Design review of the part built by this model. Coordinates are the model's own, in mm. Coordinates: 2 decimals unless noted, no trailing zeros. Order: outer loops, then holes, each group sorted by start corner. A loop starts at its lowest first (then second) coordinate and runs counter-clockwise, first axis right, second up. Notation, with made-up numbers: M 23,-36 L 36,-36 A10 cw 36,-22 Z; hole C 81,23.5 d6. An arc over 180 degrees is marked long. Answer in a Markdown table with one row per item.
from build123d import *

# Parameters (mm, degrees)
SKETCH_1_W          = 192
SKETCH_1_H          = 108
EXTRUDE_1_DEPTH     = 3
SKETCH_2_R          = 3
CUT_EXTRUDE_1_DEPTH = 4
FILLET_1_R          = 1


with BuildPart() as part:
    # Эскиз1 → Бобышка-Вытянуть1 (new body)
    with BuildSketch(Plane(origin=(0, 0, 0), x_dir=(1, 0, 0), z_dir=(0, 1, 0))):
        Rectangle(SKETCH_1_W, SKETCH_1_H)
    extrude(amount=EXTRUDE_1_DEPTH)

    # Эскиз2 → Вырез-Вытянуть1 (cut, through all)
    with BuildSketch(Plane(origin=(0, 3, 0), x_dir=(1, 0, 0), z_dir=(0, 1, 0))):
        with Locations((-73, 44)):
            Circle(SKETCH_2_R)
        with Locations((73, 44)):
            Circle(SKETCH_2_R)
        with Locations((-73, -44)):
            Circle(SKETCH_2_R)
        with Locations((73, -44)):
            Circle(SKETCH_2_R)
        Polygon((20.25, 45.5), (20.25, 25.5), (14.25, 25.5), (14.25, 13.5), (20.25, 13.5), (20.25, -9.5), (57.25, -9.5), (57.25, 6.5), (65.5, 6.5), (65.5, 25.5), (57.25, 25.5), (57.25, 45.5), align=None)
    extrude(amount=-CUT_EXTRUDE_1_DEPTH, mode=Mode.SUBTRACT)

    # Скругление1
    fillet_1_edges = [part.edges().sort_by_distance(p)[0] for p in [
        (20.25, 1.5, -45.5),
        (57.25, 1.5, -45.5),
        (57.25, 1.5, -25.5),
        (65.5, 1.5, -25.5),
        (65.5, 1.5, -6.5),
        (57.25, 1.5, -6.5),
        (57.25, 1.5, 9.5),
        (20.25, 1.5, 9.5),
        (20.25, 1.5, -13.5),
        (14.25, 1.5, -13.5),
        (14.25, 1.5, -25.5),
        (20.25, 1.5, -25.5),
    ]]
    fillet(fillet_1_edges, radius=FILLET_1_R)


solid = part.part
(1) Add section D-D, the plane z = -19. Give the boundary of the cut face in (x, y).
Return value:
| item | result |
|---|---|
| outline | M -96,0 L 14.25,0 L 14.25,3 L -96,3 Z; M 65.5,0 L 96,0 L 96,3 L 65.5,3 Z |
(2) For line 1 along X through (y, z) = (2, 44); line 2 along Z through (x, y) = (-73, 1.45); line 3 along X through (y, z) = (0.85, -44), list the stretches that pass through material, from the lowest coordinate up. Write a range as from..to.
Return value:
| item | result |
|---|---|
| line 1 | x = -96..-76, -70..70, 76..96 |
| line 2 | z = -54..-47, -41..41, 47..54 |
| line 3 | x = -96..-76, -70..20.25, 57.25..70, 76..96 |
(3) Add section B-B, the plane y = 2.3. Give the number of separate pieces and of enclosed holes in the cut face, and give its area (3 significant figures).
Return value:
| item | result |
|---|---|
| separate pieces | 1 |
| enclosed holes | 5 |
| area | 18,400 mm2 |
(4) Insertion check: pin 1 Ø5.5 at (x, z) = (73, 44) entering from -Y. The pin has a flat end and moves straight along its axis. Give the tip position at first contact, or say it passes through.
Return value:
| item | result |
|---|---|
| pin 1 | passes through |
(5) Add section C-C, the plane x = 28.5. Give the boundary of the cut face in (y, z), and give its area (3 significant figures).
Return value:
| item | result |
|---|---|
| outline | M 0,-54 L 3,-54 L 3,-45.5 L 0,-45.5 Z; M 0,9.5 L 3,9.5 L 3,54 L 0,54 Z |
| area | 159 mm2 |
(6) Draft analysis for pull direction X (two halves, no side actions). For faces 1 (the cylindrical face through (70.79, 1.52, 41.97)), 2 (the flat face through (-1, 0, -1)), state which applies: pulls with the +X half, pulls with the -X half, needs draft (parallel to the pull), parting line crosses it, or undercut.
Return value:
| item | result |
|---|---|
| face 1 | undercut |
| face 2 | needs draft |
(7) Add section A-A, the plane z = 44. Give the boundary of the cut face in (x, y), and give its area (3 significant figures).
Return value:
| item | result |
|---|---|
| outline | M -96,0 L -76,0 L -76,3 L -96,3 Z; M -70,0 L 70,0 L 70,3 L -70,3 Z; M 76,0 L 96,0 L 96,3 L 76,3 Z |
| area | 540 mm2 |
